The listing builds one solid part. Answer for the finished solid, in the listing's coordinates (mm). Give positions to 0.01 mm unless a question says otherwise; leave off trailing zeros. Write each loop counter-clockwise with the first axis right and the second up, starting at its lowest first coordinate (ties: lowest second). Pieces come first, ordered by that corner, then holes. Notation, with made-up numbers: (70.5, 79.25) -> (86.5, 79.25) arc R38 cw to (86.5, 118.25) -> close; hole circle Ø3 at (27, 67). An arc over 180 degrees is marked (long way). Put each result on its own line as item: value. Start each with the question number.
1) Find the intervals of material crossed by line 1 along X through (y, z) = (-27.5, 58) (3 decimals); line 2 along X through (y, z) = (-6, 215) (3 decimals); line 3 along Z through (x, y) = (-25, -27.5), in increasing order. Write a range as from..to.
2) Flat-ended cylindrical pins translate along their axes: pin 1 Ø7.5 at (x, z) = (502.5, -92.5) entering from -Y; pin 2 Ø12 at (x, y) = (301, -22.5) entering from -Z. Find the tip coordinate at first contact, or state that the pin passes through.
3) A cutting plane is placed at A-A (z = -173). Write down the section's boundary in (x, y) (3 decimals).
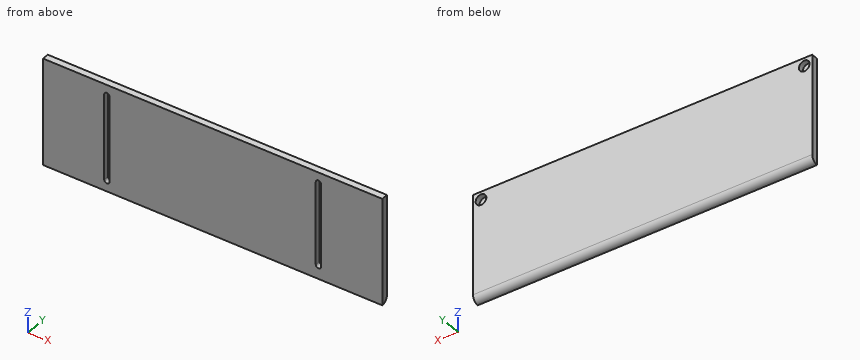
from build123d import *

# Parameters (mm, degrees)
F0_W     = 1619.25
F0_H     = 508
F1_DEPTH = 31.75
F3_DEPTH = 1619.251
F5_DEPTH = 25.4
F6_R     = 25.4
F7_DEPTH = 25.4


with BuildPart() as f1:
    # F0 (on Front) → F1 (new body)
    with BuildSketch(Plane.XZ):
        Rectangle(F0_W, F0_H)
    extrude(amount=F1_DEPTH)

    # F2 (on face) → F3 (cut, through all)
    with BuildSketch(Plane(origin=(-809.625, 0, 0), x_dir=(0, -1, 0), z_dir=(-1, 0, 0))):
        with BuildLine():
            Line((0, -222.25), (0, -254))
            Line((0, -254), (31.75, -254))
            ThreePointArc((31.75, -254), (9.29936, -244.70064), (0, -222.25))
        make_face()
    extrude(amount=-F3_DEPTH, mode=Mode.SUBTRACT)

    # F4 (on face) → F5 (cut)
    with BuildSketch(Plane.XZ.offset(31.75)):
        with BuildLine():
            Line((-492.125, -203.2), (-492.125, 203.2))
            ThreePointArc((-492.125, 203.2), (-504.825, 215.9), (-517.525, 203.2))
            Line((-517.525, 203.2), (-517.525, -203.2))
            ThreePointArc((-517.525, -203.2), (-504.825, -215.9), (-492.125, -203.2))
        make_face()
        with BuildLine():
            Line((517.525, -190.5), (517.525, 203.2))
            ThreePointArc((517.525, 203.2), (504.825, 215.9), (492.125, 203.2))
            Line((492.125, 203.2), (492.125, -190.5))
            ThreePointArc((492.125, -190.5), (504.825, -203.2), (517.525, -190.5))
        make_face()
    extrude(amount=-F5_DEPTH, mode=Mode.SUBTRACT)

    # F6 (on face) → F7 (cut)
    with BuildSketch(Plane(origin=(0, 0, 0), x_dir=(-1, 0, 0), z_dir=(0, 1, 0))):
        with Locations((-771.525, 215.9)):
            Circle(F6_R)
        with Locations((771.525, 215.9)):
            Circle(F6_R)
    extrude(amount=-F7_DEPTH, mode=Mode.SUBTRACT)


solid = f1.part
Reply:
1. line 1: x = -809.625..-517.525, -492.125..492.125, 517.525..809.625
1. line 2: x = -809.625..-796.909, -746.141..746.141, 796.909..809.625
1. line 3: z = -253.71..254
2. pin 1: stops at y = -6.35
2. pin 2: stops at z = -253.83
3. outline: (-809.625, -31.75) -> (-517.525, -31.75) -> (-517.525, -6.35) -> (-492.125, -6.35) -> (-492.125, -31.75) -> (492.125, -31.75) -> (492.125, -6.35) -> (517.525, -6.35) -> (517.525, -31.75) -> (809.625, -31.75) -> (809.625, 0) -> (-809.625, 0) -> close
